Geometry check sheet. Reference: the model listing, model coordinates, mm. Face numbers are marked on the shaded views. A direction names the side the tool comes from. Give positions to 0.01 mm unless a question says otherwise; leave off trailing zeros. Loops run counter-clockwise (first coordinate to the right, second up) from the corner with the lowest first, then second, coordinate; pieces in that order, holes last.
1. Material ranges on L1, parallel to Z at x = 11.5, y = 4.5; L2, parallel to Z at x = 4.75, y = 10; L3, parallel to Y at x = 12, z = -10, recorded low to high.
2. Cross-section at A-A, the plane z = 0. Record the cut outline in (x, y).
3. Tool access check on the marked faces 1 and 2. Record the directions out of +Z, -Z, +X, -X, +Y, -Y that give a thin tool (end or side, any length) a straight path to the whole face; none if there is none.
4. Go/stop test with flat-tipped pins: pin 1 Ø2 at (x, y) = (2.5, 58) entering from -Z; pin 2 Ø4 at (y, z) = (0.5, 61) entering from +X; pin 3 Ø9 at (y, z) = (0, 60) entering from -X. Record where each tip stops, or that it passes through.
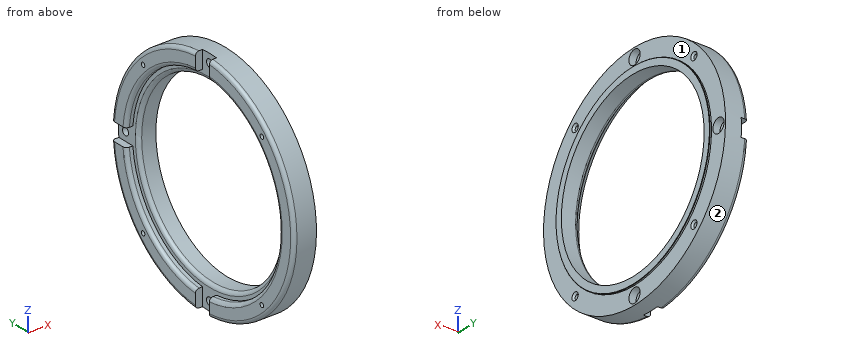
from build123d import *

# Parameters (mm, degrees)
CONG_1_R                                           = 2
ENL_V_MAT_EXTRU_1_DEPTH                            = 4
CHAMBRAGE_POUR_VIS_T_TE_HEXAGONALE_M41_D           = 4.3
CHAMBRAGE_POUR_VIS_T_TE_HEXAGONALE_M41_CBORE_D     = 8
CHAMBRAGE_POUR_VIS_T_TE_HEXAGONALE_M41_CBORE_DEPTH = 5
CHANFREIN1_SIZE                                    = 0.2
TROU_TARAUD_M31_D                                  = 2.5
TROU_TARAUD_M31_CSINK_D                            = 4.5
TROU_TARAUD_M31_CSINK_ANGLE                        = 90


with BuildPart() as part:
    # Esquisse1 → Révolution1 (revolve)
    with BuildSketch(Plane.XY, mode=Mode.PRIVATE) as r_volution1_sk:
        Polygon((0, 55), (0, 65), (13, 65), (13, 55), (14, 55), (14, 51), (4, 51), (4, 55), align=None)
    revolve(r_volution1_sk.sketch.rotate(Axis((0, 0, 0), (1, 0, 0)), 90), axis=Axis((0, 0, 0), (1, 0, 0)))

    # Congé1
    cong_1_edges = [part.edges().sort_by_distance(p)[0] for p in [
        (4, 0, -51),
        (0, 0, -65),
        (0, 0, -55),
    ]]
    fillet(cong_1_edges, radius=CONG_1_R)

    # Esquisse5 → Enlèv. mat.-Extru.1 (cut)
    with BuildSketch(Plane.ZY):
        Polygon((-5, 80), (-5, 5), (-80, 5), (-80, -5), (-5, -5), (5, -5), (80, -5), (80, 5), (5, 5), (5, 80), align=None)
    extrude(amount=-ENL_V_MAT_EXTRU_1_DEPTH, mode=Mode.SUBTRACT)

    # Chambrage pour vis à tête hexagonale M41 (through all)
    with Locations(Plane(origin=(14, 0, 0), x_dir=(0, 0, -1), z_dir=(1, 0, 0))):
        with Locations((60, 0), (-60, 0), (0, 60)):
            CounterBoreHole(CHAMBRAGE_POUR_VIS_T_TE_HEXAGONALE_M41_D / 2, CHAMBRAGE_POUR_VIS_T_TE_HEXAGONALE_M41_CBORE_D / 2, CHAMBRAGE_POUR_VIS_T_TE_HEXAGONALE_M41_CBORE_DEPTH)

    # Chanfrein1
    chanfrein1_edges = [part.edges().sort_by_distance(p)[0] for p in [
        (14, 0, -55),
    ]]
    chamfer(chanfrein1_edges, length=CHANFREIN1_SIZE)

    # Trou taraudé M31 (through all)
    with Locations(Plane(origin=(13, 0, 0), x_dir=(0, 0, -1), z_dir=(1, 0, 0))):
        with Locations((-42.426406871, 42.426406871), (42.426406871, 42.426406871), (42.426406871, -42.426406871), (-42.426406871, -42.426406871)):
            CounterSinkHole(TROU_TARAUD_M31_D / 2, TROU_TARAUD_M31_CSINK_D / 2, counter_sink_angle=TROU_TARAUD_M31_CSINK_ANGLE)


solid = part.part
Result:
1. L1: z = -64.84 to -50.8, 50.8 to 64.84
1. L2: z = -64.23 to -50.46, 50.46 to 64.23
1. L3: y = -64.23 to -50.01, 50.01 to 64.23
2. outline: (0, -63) arc R2 ccw to (2, -65) - (13, -65) - (13, -55) - (13.8, -55) - (14, -54.8) - (14, -51) - (6, -51) arc R2 ccw to (4, -53) - (4, -55) - (2, -55) arc R2 ccw to (0, -57) - close; (4, 53) arc R2 ccw to (6, 51) - (14, 51) - (14, 54.8) - (13.8, 55) - (13, 55) - (13, 56) - (9, 56) - (9, 57.85) - (4, 57.85) - close; (4, 62.15) - (9, 62.15) - (9, 64) - (13, 64) - (13, 65) - (4, 65) - close
3. face 1: +X
3. face 2: +X, -X
4. pin 1: stops at z = -31.24
4. pin 2: stops at x = 9
4. pin 3: stops at x = 4
